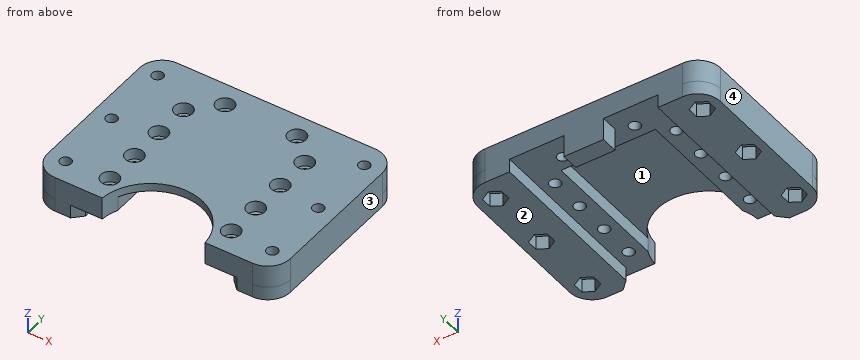
from build123d import *

# Parameters (mm, degrees)
SZKIC1_W                    = 34
SZKIC1_H                    = 40
DODANIE_WYCI_GNI_CIE1_DEPTH = 5
SZKIC2_R                    = 1.25
WYTNIJ_WYCI_GNI_CIE1_DEPTH  = 5
SZKIC3_R                    = 11.5
WYTNIJ_WYCI_GNI_CIE2_DEPTH  = 5
SZKIC4_R                    = 2
WYTNIJ_WYCI_GNI_CIE3_DEPTH  = 2.5
SZKIC5_W                    = 21
SZKIC5_H                    = 30
WYTNIJ_WYCI_GNI_CIE4_DEPTH  = 3.2
SZKIC6_W                    = 10
SZKIC6_H                    = 40
SZKIC6_R                    = 1.25
DODANIE_WYCI_GNI_CIE2_DEPTH = 5
ZAOKR_GLENIE1_R             = 5
ZAOKR_GLENIE1_OF_LUSTRO2_R  = 5
SZKIC7_W                    = 8.8
SZKIC7_H                    = 3.8
DODANIE_WYCI_GNI_CIE3_DEPTH = 5
SZKIC8_R                    = 1.25
DODANIE_WYCI_GNI_CIE4_DEPTH = 3
WYTNIJ_WYCI_GNI_CIE5_DEPTH  = 3
SZYK_LINIOWY1_COUNT         = 2
SZYK_LINIOWY1_PITCH         = 46
SZYK_LINIOWY1_COUNT_DIR2    = 3
SZYK_LINIOWY1_PITCH_DIR2    = 15
SFAZOWANIE1_SIZE            = 2


with BuildPart() as part:
    # Szkic1 → Dodanie-wyciągnięcie1 (new body)
    with BuildSketch(Plane.XY):
        Rectangle(SZKIC1_W, SZKIC1_H)
    extrude(amount=DODANIE_WYCI_GNI_CIE1_DEPTH)

    # Szkic2 → Wytnij-wyciągnięcie1 (cut)
    with BuildSketch(Plane.XY.offset(5)):
        with Locations((8, 15)):
            Circle(SZKIC2_R)
        with Locations((13.5, 9.5)):
            Circle(SZKIC2_R)
        with Locations((13.5, 1.5)):
            Circle(SZKIC2_R)
        with Locations((13.5, -6.5)):
            Circle(SZKIC2_R)
        with Locations((13.5, -14.5)):
            Circle(SZKIC2_R)
    wytnij_wyci_gni_cie1 = extrude(amount=-WYTNIJ_WYCI_GNI_CIE1_DEPTH, mode=Mode.SUBTRACT)

    # Szkic3 → Wytnij-wyciągnięcie2 (cut)
    with BuildSketch(Plane.XY.offset(5)):
        with Locations((0, -21)):
            Circle(SZKIC3_R)
    extrude(amount=-WYTNIJ_WYCI_GNI_CIE2_DEPTH, mode=Mode.SUBTRACT)

    # Szkic4 → Wytnij-wyciągnięcie3 (cut)
    with BuildSketch(Plane.XY.offset(5)):
        with Locations((8, 15)):
            Circle(SZKIC4_R)
        with Locations((13.5, 9.5)):
            Circle(SZKIC4_R)
        with Locations((13.5, 1.5)):
            Circle(SZKIC4_R)
        with Locations((13.5, -6.5)):
            Circle(SZKIC4_R)
        with Locations((13.5, -14.5)):
            Circle(SZKIC4_R)
    wytnij_wyci_gni_cie3 = extrude(amount=-WYTNIJ_WYCI_GNI_CIE3_DEPTH, mode=Mode.SUBTRACT)

    # Lustro1: Wytnij-wyciągnięcie1, Wytnij-wyciągnięcie3 across plane
    add(wytnij_wyci_gni_cie1.mirror(Plane(origin=(0, 0, 0), x_dir=(0, 0, 1), z_dir=(1, 0, 0))), mode=Mode.SUBTRACT)
    add(wytnij_wyci_gni_cie3.mirror(Plane(origin=(0, 0, 0), x_dir=(0, 0, 1), z_dir=(1, 0, 0))), mode=Mode.SUBTRACT)

    # Szkic5 → Wytnij-wyciągnięcie4 (cut)
    with BuildSketch(Plane(origin=(0, 0, 0), x_dir=(-1, 0, 0), z_dir=(0, 0, -1))):
        with Locations((0, -3)):
            Rectangle(SZKIC5_W, SZKIC5_H)
    extrude(amount=-WYTNIJ_WYCI_GNI_CIE4_DEPTH, mode=Mode.SUBTRACT)

    # Szkic6 → Dodanie-wyciągnięcie2 (add)
    with BuildSketch(Plane.XY.offset(5)):
        with Locations((-22, 0)):
            Rectangle(SZKIC6_W, SZKIC6_H)
        with Locations((-23, -15)):
            Circle(SZKIC6_R, mode=Mode.SUBTRACT)
        with Locations((-23, 0)):
            Circle(SZKIC6_R, mode=Mode.SUBTRACT)
        with Locations((-23, 15)):
            Circle(SZKIC6_R, mode=Mode.SUBTRACT)
    dodanie_wyci_gni_cie2 = extrude(amount=-DODANIE_WYCI_GNI_CIE2_DEPTH)

    # Zaokrąglenie1
    zaokr_glenie1_edges = [part.edges().sort_by_distance(p)[0] for p in [
        (-27, -20, 2.5),
        (-27, 20, 2.5),
    ]]
    fillet(zaokr_glenie1_edges, radius=ZAOKR_GLENIE1_R)

    # Lustro2: Dodanie-wyciągnięcie2 across plane
    add(dodanie_wyci_gni_cie2.mirror(Plane(origin=(0, 0, 0), x_dir=(0, 0, 1), z_dir=(1, 0, 0))))

    # Zaokrąglenie1 of Lustro2
    zaokr_glenie1_of_lustro2_edges = [part.edges().sort_by_distance(p)[0] for p in [
        (27, -20, 2.5),
        (27, 20, 2.5),
    ]]
    fillet(zaokr_glenie1_of_lustro2_edges, radius=ZAOKR_GLENIE1_OF_LUSTRO2_R)

    # Szkic7 → Dodanie-wyciągnięcie3 (add)
    with BuildSketch(Plane(origin=(0, 0, 0), x_dir=(-1, 0, 0), z_dir=(0, 0, -1))):
        with Locations((0, 18.1)):
            Rectangle(SZKIC7_W, SZKIC7_H)
    extrude(amount=DODANIE_WYCI_GNI_CIE3_DEPTH)

    # Szkic8 → Dodanie-wyciągnięcie4 (add)
    # profile 1 of 2: a face of its own
    with BuildSketch(Plane(origin=(0, 0, 0), x_dir=(-1, 0, 0), z_dir=(0, 0, -1))):
        with BuildLine():
            Line((-16.5, -20), (-16.5, 20))
            Line((-16.5, 20), (-22, 20))
            ThreePointArc((-22, 20), (-25.535533906, 18.535533906), (-27, 15))
            Line((-27, 15), (-27, -15))
            ThreePointArc((-27, -15), (-25.535533906, -18.535533906), (-22, -20))
            Line((-22, -20), (-16.5, -20))
        make_face()
        with Locations(Location((-23, -15, 0), (0, 0, 180))):
            Circle(SZKIC8_R, mode=Mode.SUBTRACT)
        with Locations(Location((-23, 0, 0), (0, 0, 180))):
            Circle(SZKIC8_R, mode=Mode.SUBTRACT)
        with Locations(Location((-23, 15, 0), (0, 0, 180))):
            Circle(SZKIC8_R, mode=Mode.SUBTRACT)
    # profile 2 of 2: a face of its own
    with BuildSketch(Plane(origin=(0, 0, 0), x_dir=(-1, 0, 0), z_dir=(0, 0, -1))):
        with BuildLine():
            Line((22, 20), (16.5, 20))
            Line((16.5, 20), (16.5, -20))
            Line((16.5, -20), (22, -20))
            ThreePointArc((22, -20), (25.535533906, -18.535533906), (27, -15))
            Line((27, -15), (27, 15))
            ThreePointArc((27, 15), (25.535533906, 18.535533906), (22, 20))
        make_face()
        with Locations(Location((23, -15, 0), (0, 0, 180))):
            Circle(SZKIC8_R, mode=Mode.SUBTRACT)
        with Locations(Location((23, 0, 0), (0, 0, 180))):
            Circle(SZKIC8_R, mode=Mode.SUBTRACT)
        with Locations(Location((23, 15, 0), (0, 0, 180))):
            Circle(SZKIC8_R, mode=Mode.SUBTRACT)
    extrude(amount=DODANIE_WYCI_GNI_CIE4_DEPTH)

    # Szkic9 → Wytnij-wyciągnięcie5 (cut)
    with BuildSketch(Plane(origin=(0, 0, -3), x_dir=(-1, 0, 0), z_dir=(0, 0, -1))):
        Polygon((-23, 12.575128869), (-20.9, 13.787564435), (-20.9, 16.212435565), (-23, 17.424871131), (-25.1, 16.212435565), (-25.1, 13.787564435), align=None)
    wytnij_wyci_gni_cie5 = extrude(amount=-WYTNIJ_WYCI_GNI_CIE5_DEPTH, mode=Mode.SUBTRACT)

    # Szyk liniowy1: Wytnij-wyci_gni_cie5 2 × 3
    with Locations(*[(-i * SZYK_LINIOWY1_PITCH, -j * SZYK_LINIOWY1_PITCH_DIR2, 0) for i in range(SZYK_LINIOWY1_COUNT) for j in range(SZYK_LINIOWY1_COUNT_DIR2) if (i, j) != (0, 0)]):
        add(wytnij_wyci_gni_cie5, mode=Mode.SUBTRACT)

    # Sfazowanie1
    sfazowanie1_edges = [part.edges().sort_by_distance(p)[0] for p in [
        (16.5, -20, -1.5),
        (-16.5, -20, -1.5),
    ]]
    chamfer(sfazowanie1_edges, length=SFAZOWANIE1_SIZE)


solid = part.part
Verification items for the finished model (mm, model axes). Face numbers are marked on the shaded views. Round coordinates to 2 decimals unless told otherwise and drop trailing zeros. Loops run counter-clockwise (first coordinate to the right, second up) from the corner with the lowest first, then second, coordinate; pieces in that order, holes last. Notation, with made-up numbers: (-33, -13.5) - (-28, -13.5) arc R18 ccw to (-28, 7.5) - close; hole circle Ø10 at (-39.75, -19). An arc over 180 degrees is marked (long way). Use a Markdown table: item, result. Add a question column.
1. Section check A-A, the plane y = 9.5. Record the boundary of the cut face in (x, z).
2. Gauge pin test, flat ends, axial feed: pin 1 (6 mm diameter, centred on x = 6, y = 2.5, fed in from -Z); pin 2 (3 mm diameter, centred on x = 8, y = 15, fed in from -Z); pin 3 (1.5 mm diameter, centred on x = 16, y = -16, fed in from -Z). Record the tip position at first contact, or that the pin passes through.
3. Section check C-C, the plane x = 8. Record the boundary of the cut face in (y, z), plus the area to 3 significant figures.
4. Release check for a two-part mould opening along X. For the marked faces 1, 2, 3 and 4 record: released by +X, released by -X, zero draft, split by the parting line, or undercut.
5. Section check D-D, the plane y = -3. Record the boundary of the cut face in (x, z).
6. Section check B-B, the plane z = -1.5. Give the number of separate pieces and of enclosed holes in the cut face, plus the area to 3 significant figures.
7. Thickness scan on probe 1 along Y at (x, z) = (13.5, 0.7); probe 2 along Y at (x, z) = (13.5, 4.15); probe 3 along Y at (x, z) = (-23, 2.65). Record the ranges inside material, lowest first. Write a range as [from, to].
Checks:
| question | item | result |
|---|---|---|
| 1 | outline | (-27, -3) - (-16.5, -3) - (-16.5, 0) - (-14.75, 0) - (-14.75, 2.5) - (-15.5, 2.5) - (-15.5, 5) - (-27, 5) - close; (-12.25, 0) - (-10.5, 0) - (-10.5, 3.2) - (10.5, 3.2) - (10.5, 0) - (12.25, 0) - (12.25, 2.5) - (11.5, 2.5) - (11.5, 5) - (-11.5, 5) - (-11.5, 2.5) - (-12.25, 2.5) - close; (14.75, 0) - (16.5, 0) - (16.5, -3) - (27, -3) - (27, 5) - (15.5, 5) - (15.5, 2.5) - (14.75, 2.5) - close |
| 2 | pin 1 | stops at z = 3.2 |
| 2 | pin 2 | stops at z = 0 |
| 2 | pin 3 | stops at z = -3 |
| 3 | outline | (-12.74, 3.2) - (12, 3.2) - (12, 0) - (13.75, 0) - (13.75, 2.5) - (13, 2.5) - (13, 5) - (-12.74, 5) - close; (16.25, 0) - (20, 0) - (20, 5) - (17, 5) - (17, 2.5) - (16.25, 2.5) - close |
| 3 | area | 68.3 mm^2 |
| 4 | face 1 | undercut |
| 4 | face 2 | zero draft |
| 4 | face 3 | released by +X |
| 4 | face 4 | released by -X |
| 5 | outline | (-27, -3) - (-16.5, -3) - (-16.5, 0) - (-10.5, 0) - (-10.5, 3.2) - (10.5, 3.2) - (10.5, 0) - (16.5, 0) - (16.5, -3) - (27, -3) - (27, 5) - (-27, 5) - close |
| 6 | separate pieces | 3 |
| 6 | enclosed holes | 6 |
| 6 | area | 756 mm^2 |
| 7 | probe 1 | y = [-20, -15.75], [-13.25, -7.75], [-5.25, 0.25], [2.75, 8.25], [10.75, 20] |
| 7 | probe 2 | y = [-20, -16.5], [-12.5, -8.5], [-4.5, -0.5], [3.5, 7.5], [11.5, 20] |
| 7 | probe 3 | y = [-19.9, -16.25], [-13.75, -1.25], [1.25, 13.75], [16.25, 19.9] |
